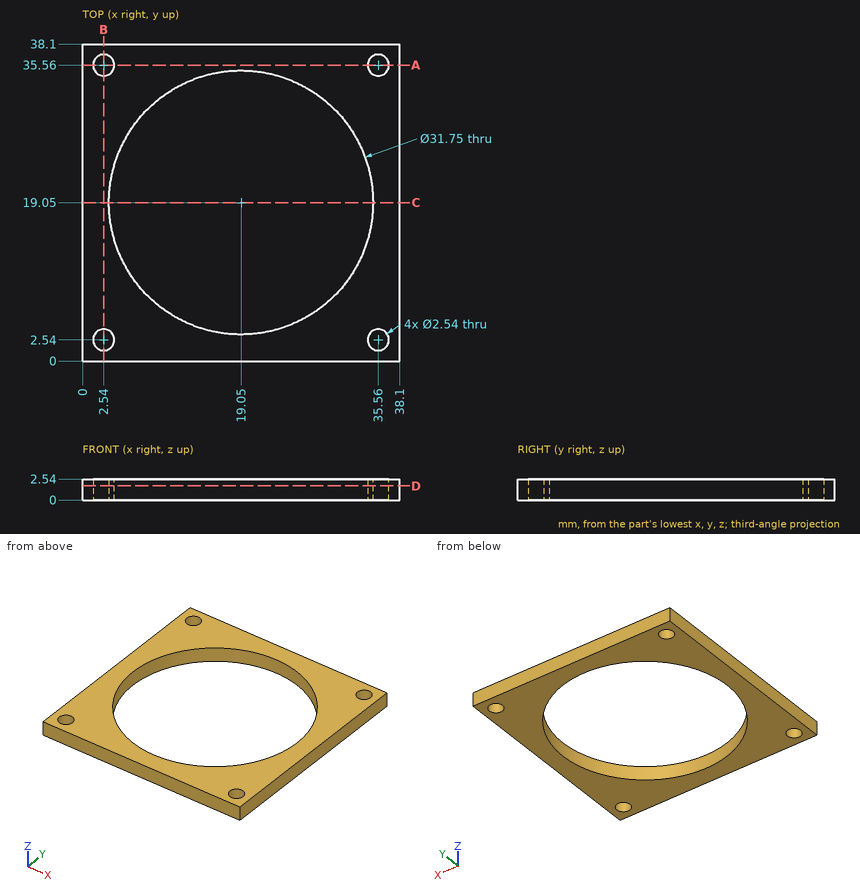
Check sheet for the drawn part. Datum: minimum x, y, z corner. Units: mm. Give positions to 0.01 mm unless a question says otherwise; leave off trailing zeros. Order: outer loops, then holes, each group sorted by start corner. A loop starts at its lowest first (then second) coordinate and runs counter-clockwise, first axis right, second up. Notation, with made-up numbers: (55.25, 62) - (100.25, 62) arc R19 cw to (100.25, 88) - close; hole circle Ø6 at (85.25, -39). An arc over 180 degrees is marked (long way). Write item = value, one per line. Start each with the question number.
1) Section check C-C (y = 19.05). Enter the section's corners in (x, z) (3 decimals), then the cut area to 3 significant figures.
2) Scan lines: L1, parallel to X at y = 35.56, z = 1.2; L2, parallel to Y at x = 19.05, z = 0.8 (3 decimals). Record each from-to range of solid material in increasing order.
3) Section check A-A (y = 35.56). Enter the section's corners in (x, z).
4) Section check D-D (z = 1.7). Enter the section's corners in (x, y) (3 decimals).
Geometry check:
q1.outline = (0, 0) - (3.175, 0) - (3.175, 2.54) - (0, 2.54) - close; (34.925, 0) - (38.1, 0) - (38.1, 2.54) - (34.925, 2.54) - close
q1.area = 16.1 mm2
q2.L1 = 0 to 1.27, 3.81 to 34.29, 36.83 to 38.1
q2.L2 = 0 to 3.175, 34.925 to 38.1
q3.outline = (0, 0) - (1.27, 0) - (1.27, 2.54) - (0, 2.54) - close; (3.81, 0) - (34.29, 0) - (34.29, 2.54) - (3.81, 2.54) - close; (36.83, 0) - (38.1, 0) - (38.1, 2.54) - (36.83, 2.54) - close
q4.outline = (0, 0) - (38.1, 0) - (38.1, 38.1) - (0, 38.1) - close; hole circle Ø2.54 at (2.54, 2.54); hole circle Ø2.54 at (2.54, 35.56); hole circle Ø31.75 at (19.05, 19.05); hole circle Ø2.54 at (35.56, 2.54); hole circle Ø2.54 at (35.56, 35.56)
